from build123d import *

# Parameters (mm, degrees)
F0_R     = 25
F1_DEPTH = 88
F2_W     = 88
F2_H     = 40
F3_DEPTH = 50
F5_DEPTH = 16
F7_DEPTH = 9


with BuildPart() as f1:
    # F0 (on Top) → F1 (new body)
    with BuildSketch(Plane.XY):
        with BuildLine():
            Line((0, 75), (0, 0))
            Line((0, 0), (50, 0))
            ThreePointArc((50, 0), (87.5, 37.5), (50, 75))
            Line((50, 75), (0, 75))
        make_face()
        with Locations((50, 37.5)):
            Circle(F0_R, mode=Mode.SUBTRACT)
    extrude(amount=F1_DEPTH)

    # F2 (on Right) → F3 (join)
    with BuildSketch(Plane.YZ):
        with Locations((-44, 20)):
            Rectangle(F2_W, F2_H)
        with BuildLine():
            ThreePointArc((-14, 20), (-17.2218254069, 12.2218254069), (-25, 9))
            Line((-25, 9), (-63, 9))
            ThreePointArc((-63, 9), (-74, 20), (-63, 31))
            Line((-63, 31), (-25, 31))
            ThreePointArc((-25, 31), (-17.2218254069, 27.7781745931), (-14, 20))
        make_face(mode=Mode.SUBTRACT)
    extrude(amount=F3_DEPTH)

    # F4 (on Right) → F5 (join)
    with BuildSketch(Plane.YZ):
        Polygon((-88, 40), (0, 40), (0, 88), align=None)
    extrude(amount=F5_DEPTH)

    # F6 (on face) → F7 (cut, through all)
    with BuildSketch(Plane.XY.offset(40)):
        with BuildLine():
            ThreePointArc((33, -38), (28.7573593129, -48.2426406871), (39, -44))
            ThreePointArc((39, -44), (37.2426406871, -39.7573593129), (33, -38))
        make_face()
    extrude(amount=-F7_DEPTH, mode=Mode.SUBTRACT)


solid = f1.part
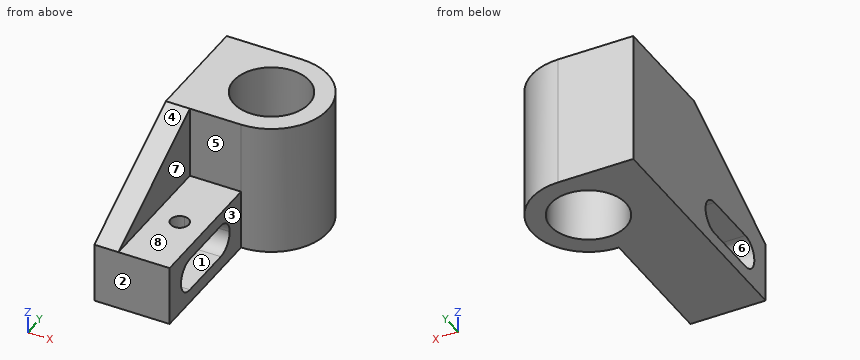
Model file for the job. Use its own axes, mm. Face numbers are marked on the shaded views. A direction names the side the tool comes from. Give positions to 0.01 mm unless a question says otherwise; leave off trailing zeros. Order: outer loops, then holes, each group sorted by start corner. A loop starts at its lowest first (then second) coordinate and runs counter-clockwise, first axis right, second up. Notation, with made-up numbers: M 0.25,84 L 24.25,84 A20 ccw 24.25,93 Z; hole C 34,-19.5 d7. An arc over 180 degrees is marked long. Put each result on its own line as item: value. Start each with the question number.
(1) Band-saw the part on C-C on y = 32.5. Give the cut face in (x, z), then the cut area to 3 significant figures.
(2) Band-saw the part on D-D on y = -47. Give the cut face in (x, z), then the cut area to 3 significant figures.
(3) Drill centre lines: L1, parallel to X at y = -44, z = 38; L2, parallel to Z at x = 37, y = -54.5; L3, parallel to Y at x = 50, z = 55. Where is each one in solid material? Low to high. Write a range as [from, to].
(4) Band-saw the part on A-A on z = 82. Give the cut face in (x, y), then the cut area to 3 significant figures.
(5) Pull direction Z, two halves, no side cores. Call the marked faces 6, 7 and 8: released by +Z, released by -Z, zero draft, split by the parting line, or undercut.
(6) Tool access for the marked faces 1, 2, 3, 4 and 5: list every direction of +Z, -Z, +X, -X, +Y, -Y with a clear straight run to the whole face (end or side of a thin tool).
(7) Band-saw the part on B-B on x = 22.5. Give the cut face in (y, z), then the cut area to 3 significant figures.
(8) Pin check, flat tips, straight feed: pin 1 Ø10 at (x, z) = (61.5, 58) entering from -Y; pin 2 Ø12 at (x, z) = (65.5, 53.5) entering from -Y; pin 3 Ø2 at (x, y) = (28.5, -16) entering from +Z. Stop position of each tip, or through.
Results below:
1. outline: M 0,0 L 25.51,0 L 25.51,88 L 0,88 Z; M 74.49,0 L 87.17,0 L 87.17,88 L 74.49,88 Z
1. area: 3,360 mm2
2. outline: M 0,0 L 50,0 L 50,9 L 0,9 Z; M 0,31 L 27.8,31 L 27.8,40 L 16,40 L 16,62.36 L 0,62.36 Z; M 38.2,31 L 50,31 L 50,40 L 38.2,40 Z
2. area: 1,160 mm2
3. L1: x = [0, 27], [39, 50]
3. L2: z = [0, 9], [31, 40]
3. L3: y = [0, 12.5], [62.5, 75]
4. outline: M 0,-11 L 16,-11 L 16,0 L 50,0 A37.5 ccw 50,75 L 0,75 Z; hole C 50,37.5 d50
4. area: 4,170 mm2
5. face 6: undercut
5. face 7: zero draft
5. face 8: released by +Z
6. face 1: +X, -X
6. face 2: +Z, -Z, +X, -X, -Y
6. face 3: +Z, -Z, +X, -Y
6. face 4: +Z, +X, -X, -Y
6. face 5: +Z, +X, -Y
7. outline: M -88,0 L 75,0 L 75,88 L 0,88 L 0,40 L -88,40 Z; hole M -63,9 L -25,9 A11 ccw -25,31 L -63,31 A11 ccw Z
7. area: 8,900 mm2
8. pin 1: stops at y = 0.57
8. pin 2: stops at y = 1.22
8. pin 3: stops at z = 40
